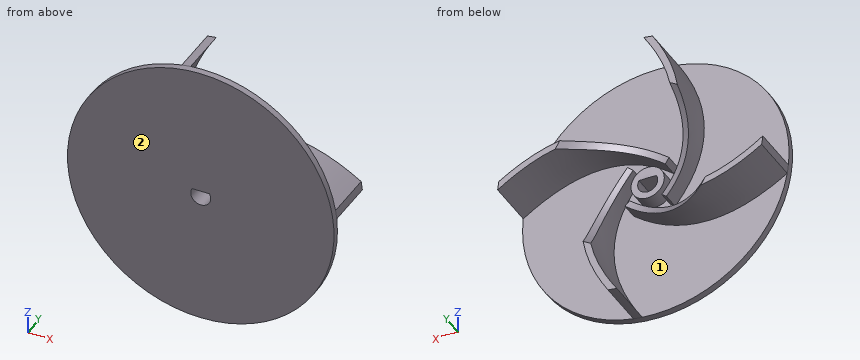
```python
from build123d import *

# Parameters (mm, degrees)
SKETCH1_R           = 40
BOSS_EXTRUDE1_DEPTH = 2
SKETCH2_R           = 5
BOSS_EXTRUDE2_DEPTH = 7
CUT_EXTRUDE2_DEPTH  = 58
BOSS_EXTRUDE4_DEPTH = 15
CIRPATTERN1_COUNT   = 4


# Read off the part's stored shape, not the designer's step: Boss-Extrude4
with BuildPart() as part:
    # Sketch1 → Boss-Extrude1 (new body)
    with BuildSketch(Plane(origin=(0, 0, 0), x_dir=(1, 0, 0), z_dir=(0, 1, 0))):
        with Locations(Location((0, 0, 0), (0, 0, 270))):
            Circle(SKETCH1_R)
    extrude(amount=BOSS_EXTRUDE1_DEPTH)

    # Sketch2 → Boss-Extrude2 (add)
    with BuildSketch(Plane(origin=(0, 0, 0), x_dir=(1, 0, 0), z_dir=(0, 1, 0))):
        with Locations(Location((0, 0, 0), (0, 0, 270))):
            Circle(SKETCH2_R)
    extrude(amount=BOSS_EXTRUDE2_DEPTH)

    # Sketch4 → Cut-Extrude2 (cut, through all)
    with BuildSketch(Plane(origin=(0, 0, 0), x_dir=(1, 0, 0), z_dir=(0, 1, 0))):
        with BuildLine():
            Line((-2.598076211, -1.5), (2.598076211, -1.5))
            ThreePointArc((2.598076211, -1.5), (0, 3), (-2.598076211, -1.5))
        make_face()
    extrude(amount=CUT_EXTRUDE2_DEPTH, mode=Mode.SUBTRACT)

    # Boss-Extrude4 outline → Boss-Extrude4 (add)
    with BuildSketch(Plane(origin=(0, 2, 0), x_dir=(1, 0, 0), z_dir=(0, 1, 0))):
        with BuildLine():
            Line((5.360007285, 4.288004046), (6.620393902, 5.840880595))
            add(Edge.make_bspline(
                [(6.620393902, 5.840880595), (4.446591581, 7.60523936), (-2.240614046, 11.838382972), (-11.595270921, 14.60910996), (-21.325153615, 14.461577349), (-32.769869479, 10.987725064), (-39.434498844, 6.70226088)],
                knots=[0, 0, 0, 0.0625, 0.1875, 0.3125, 0.4375, 0.597789977, 0.597789977, 0.597789977], degree=2))
            ThreePointArc((-39.434498844, 6.70226088), (-39.635737327, 5.385937855), (-39.793049423, 4.063645853))
            add(Edge.make_bspline(
                [(5.360007285, 4.288004046), (3.271766893, 5.982916783), (-3.097296011, 10.009630326), (-11.871370928, 12.604159995), (-20.990596912, 12.469062744), (-32.556083101, 8.970033013), (-39.793049423, 4.063645853)],
                knots=[0, 0, 0, 0.0625, 0.1875, 0.3125, 0.4375, 0.615564575, 0.615564575, 0.615564575], degree=2))
        make_face()
    boss_extrude4 = extrude(amount=BOSS_EXTRUDE4_DEPTH)

    # CirPattern1: Boss-Extrude4 ×4 about axis
    cirpattern1_axis = Axis((0, 7, 0), (0, 1, 0))
    for i in range(1, CIRPATTERN1_COUNT):
        add(boss_extrude4.rotate(cirpattern1_axis, i * 360 / CIRPATTERN1_COUNT))

    # Sketch6 → Cut-Revolve1 (revolve, cut)
    with BuildSketch(Plane.XY, mode=Mode.PRIVATE) as cut_revolve1_sk:
        with BuildLine():
            Line((0, 7), (0, 17))
            Line((0, 17), (-25.416272602, 17))
            add(Edge.make_bspline(
                [(0, 7), (-15.082792744, 5.256181573), (-25.416272602, 17)],
                knots=[0, 0, 0, 1, 1, 1], degree=2))
        make_face()
    revolve(cut_revolve1_sk.sketch.rotate(Axis((0, 7, 0), (0, 1, 0)), 270), axis=Axis((0, 7, 0), (0, 1, 0)), mode=Mode.SUBTRACT)


solid = part.part
```
For this review, take the finished solid that the model builds, in its own axes (mm). Face numbers are marked on the shaded views. Coordinates: 2 decimals unless noted, no trailing zeros. Use CSV: the item, a comma, the result in double quotes. Start each with the question number.
Item 1: Wall thickness on probe 1 along X at (y, z) = (3, 0); probe 2 along Z at (x, y) = (0, 4.25); probe 3 along Y at (x, z) = (-22, 20): over which ranges is each line inside the solid? List them lowest first.
Item 2: Draft analysis for pull direction X (two halves, no side actions). For the marked faces 1 and 2, state which applies: pulls with the +X half, pulls with the -X half, needs draft (parallel to the pull), parting line crosses it, or undercut.
Item 3: Insertion check: pin 1 (1 mm diameter, centred on y = 11.5, z = -16.5, fed in from -X); pin 2 (10 mm diameter, centred on x = 22, y = 4, fed in from -Z); pin 3 (1 mm diameter, centred on y = 11.5, z = 19, fed in from -X). Each pin has a flat end and moves straight along its axis. Give the tip position at first contact, or say it passes through.
Item 4: We need section A-A, the plane y = 3.75. Give the number of separate pieces and of enclosed holes in the cut face, then the cut area to 3 significant figures.
Derived:
1,probe 1,"x = -10.32 to -8.02, -5 to -3, 3 to 5, 8.02 to 10.32"
1,probe 2,"z = -10.32 to -8.02, -5 to -3, 1.5 to 5, 8.02 to 10.32"
1,probe 3,"y = 0 to 2"
2,face 1,"undercut"
2,face 2,"needs draft"
3,pin 1,"stops at x = 12.52"
3,pin 2,"stops at z = -36.01"
3,pin 3,"stops at x = -14.44"
4,separate pieces,"5"
4,enclosed holes,"1"
4,area,"451 mm^2"
